Geometry: final body of the model. Coordinates: model frame, mm. A direction names the side the tool comes from. Round coordinates to 2 decimals unless told otherwise and drop trailing zeros. Write each loop counter-clockwise with the first axis right and the second up, starting at its lowest first coordinate (ties: lowest second). Pieces come first, ordered by that corner, then holes. Notation, with made-up numbers: M 12,31.25 L 58,31.25 A14 cw 58,52.25 Z; hole C 16,2.25 d10. An arc over 180 degrees is marked long. Answer as CSV lines item,"result". Start each with the question number.
Q1. Ray query, probe 1 along X at (y, z) = (-17.5, -7.5); probe 2 along Y at (x, z) = (-13, 0.35). Return the intervals inside material, ascending.
Q2. Section query C-C on y = -9.5. Output: boundary loops of the cut face in (x, z), and give its area (3 significant figures).
Q3. Section query A-A on x = -13. Output: boundary loops of the cut face in (y, z).
Q4. Mould query, pull axis Y, two halves, no side actions, for faces 1 (the flat face through (-1.9, -23.2, -9.4)), 2 (the cylindrical face through (-19.265, -7.155, -0.008)), 3 (the flat face through (0, -24.2, -4)), 4 (the flat face through (-21, -22, -6.3)). Classes: pulls with the +Y half, pulls with the -Y half, needs draft (parallel to the pull), parting line crosses it, or undercut.
Q5. Reachability of faces 5 (the flat face through (0, 6, 0.6)), 6 (the cylindrical face through (21.224, -21.335, -7.04)), 7 (the flat face through (2.55, -13, 0)) from +Z, -Z, +X, -X, +Y, -Y: full face, straight path, thin tool, end or side. Return the list, or none.
Q6. Section query D-D on x = -3.5. Output: boundary loops of the cut face in (y, z), and give its area (3 significant figures).
Q7. Section query B-B on z = -2. Output: boundary loops of the cut face in (x, y).
Q8. First-contact query: pin 1 (0.6 mm diameter, centred on x = -22, y = -21.5, fed in from -Z); pin 2 (6 mm diameter, centred on x = -1.5, y = 13, fed in from -Z). Flat tips, straight axial feed; report the tip coordinate or a pass-through.
```python
from build123d import *

# Parameters (mm, degrees)
F0_W     = 23
F0_H     = 23
F0_R     = 8.5
F1_DEPTH = 0.6
F3_DEPTH = 10
F4_W     = 2.6
F4_H     = 2.6
F4_R     = 0.6
F5_DEPTH = 5.7
F6_DEPTH = 7.2


with BuildPart() as f1:
    # F0 (on Top) → F1 (new body, symmetric)
    with BuildSketch(Plane.XY):
        with Locations((-11.5, 11.5)):
            Rectangle(F0_W, F0_H)
        Polygon((0, -10.1312079445), (0, 0), (-23, 0), (-23, -23), (0, -23), (0, -15.2312079445), (-2.55, -15.2312079445), (-2.55, -10.1312079445), align=None)
        with Locations((-13, -12.9)):
            Circle(F0_R, mode=Mode.SUBTRACT)
        with Locations((11.5, 11.5)):
            Rectangle(F0_W, F0_H)
        Polygon((23, 0), (0, 0), (0, -10.1312079445), (2.55, -10.1312079445), (2.55, -15.2312079445), (0, -15.2312079445), (0, -23), (23, -23), align=None)
        with Locations((13, -12.9)):
            Circle(F0_R, mode=Mode.SUBTRACT)
    extrude(amount=F1_DEPTH, both=True)

    # F2 (on face) → F3 (join)
    with BuildSketch(Plane.XY.offset(0.6)):
        Polygon((0, 23), (23, 23), (23, -23), (0, -23), (0, -24.2), (24.2, -24.2), (24.2, 24.2), (0, 24.2), align=None)
        Polygon((-23, 23), (0, 23), (0, 24.2), (-24.2, 24.2), (-24.2, -24.2), (0, -24.2), (0, -23), (-23, -23), align=None)
    extrude(amount=-F3_DEPTH)

    # F4 (on face) → F5 (join)
    with BuildSketch(Plane(origin=(0, 0, -0.6), x_dir=(1, 0, 0), z_dir=(0, 0, -1))):
        with Locations((21.7, 21.7)):
            Rectangle(F4_W, F4_H)
        with Locations((21.7, 21.7)):
            Circle(F4_R, mode=Mode.SUBTRACT)
        with Locations((-21.7, 21.7)):
            Rectangle(F4_W, F4_H)
        with Locations((-21.7, 21.7)):
            Circle(F4_R, mode=Mode.SUBTRACT)
        with Locations((-21.7, 4.7)):
            Rectangle(F4_W, F4_H)
        with Locations((-21.7, 4.7)):
            Circle(F4_R, mode=Mode.SUBTRACT)
        with Locations((21.7, 4.7000000451)):
            Rectangle(F4_W, F4_H)
        with Locations((21.7, 4.7000000451)):
            Circle(F4_R, mode=Mode.SUBTRACT)
    extrude(amount=F5_DEPTH)

    # F6 (add): faces of the model
    f6_faces = [f1.faces().sort_by_distance(p)[0] for p in [
        (-21.7, -4.7, -0.6),
        (-21.7, -21.7, -0.6),
        (21.7, -21.7, -0.6),
        (21.7, -4.7000000451, -0.6),
    ]]
    extrude(f6_faces, amount=F6_DEPTH)


solid = f1.part
```
Entries:
1,probe 1,"x = -24.2 to -23, 23 to 24.2"
1,probe 2,"y = -24.2 to -21.4, -4.4 to 24.2"
2,outline,"M -24.2,-9.4 L -23,-9.4 L -23,-0.6 L -20.79,-0.6 L -20.79,0.6 L -24.2,0.6 Z; M -5.21,-0.6 L 5.21,-0.6 L 5.21,0.6 L -5.21,0.6 Z; M 20.79,-0.6 L 23,-0.6 L 23,-9.4 L 24.2,-9.4 L 24.2,0.6 L 20.79,0.6 Z"
2,area,"41.8 mm^2"
3,outline,"M -24.2,-9.4 L -23,-9.4 L -23,-0.6 L -21.4,-0.6 L -21.4,0.6 L -24.2,0.6 Z; M -4.4,-0.6 L 23,-0.6 L 23,-9.4 L 24.2,-9.4 L 24.2,0.6 L -4.4,0.6 Z"
4,face 1,"needs draft"
4,face 2,"undercut"
4,face 3,"pulls with the -Y half"
4,face 4,"undercut"
5,face 5,"+Z, +X, -X, +Y, -Y"
5,face 6,"-Z"
5,face 7,"+Z, -Z"
6,outline,"M -24.2,-9.4 L -23,-9.4 L -23,-0.6 L 23,-0.6 L 23,-9.4 L 24.2,-9.4 L 24.2,0.6 L -24.2,0.6 Z"
6,area,"79.2 mm^2"
7,outline,"M -24.2,-24.2 L 24.2,-24.2 L 24.2,24.2 L -24.2,24.2 Z; hole M -23,-20.4 L -20.4,-20.4 L -20.4,-23 L 20.4,-23 L 20.4,-20.4 L 23,-20.4 L 23,-6 L 20.4,-6 L 20.4,-3.4 L 23,-3.4 L 23,23 L -23,23 L -23,-3.4 L -20.4,-3.4 L -20.4,-6 L -23,-6 Z"
8,pin 1,"stops at z = -7.8"
8,pin 2,"stops at z = -0.6"
